Autodesk Fusion 360 part; units mm, degrees
sketch "Sketch1" plane through (0, 0, 0) normal (0, 0, 1) x (1, 0, 0)
  circle A0 centre (0, 0) radius 1.65
  circle A1 centre (0, 0) radius 3.65
  line L0 (0, 0) -> (0, -3.65)
  line L1 (0, 0) -> (0, 3.65)
  line L2 (0, 3.65) -> (15, 3.65)
  line L3 (0, -3.65) -> (15, -3.65)
  line L4 (0, 1.65) -> (12.4019, 1.65)
  line L5 (0, -1.65) -> (12.4019, -1.65)
  line L6 (16.5, 2.15) -> (16.5, 1.65)
  line L7 (16.5, -2.15) -> (16.5, -1.65)
  arc A2 (15, -0.15) -> (13.701, -0.9) centre (15, -1.65) ccw
  arc A3 (16.5, -1.65) -> (15, -0.15) centre (15, -1.65) ccw
  arc A4 (13.701, 0.9) -> (15, 0.15) centre (15, 1.65) ccw
  arc A5 (15, 0.15) -> (16.5, 1.65) centre (15, 1.65) ccw
  arc A6 (13.701, 0.9) -> (12.4019, 1.65) centre (12.4019, 0.15) ccw
  arc A7 (12.4019, -1.65) -> (13.701, -0.9) centre (12.4019, -0.15) ccw
  arc A8 (15, -3.65) -> (16.5, -2.15) centre (15, -2.15) ccw
  arc A9 (16.5, 2.15) -> (15, 3.65) centre (15, 2.15) ccw
  point P0 (16.5, 3.65)
  point P1 (16.5, -3.65)
  point P2 (13.5, 1.65)
  point P3 (13.5, -1.65)
  point P4 (16.5, 3.65)
  point P5 (16.5, 0.15)
  point P6 (16.5, -3.65)
  point P7 (16.5, -0.15)
  point P8 (13.5, 0.15)
  point P9 (13.5, -0.15)
  dimension "d1" = 3.3
  dimension "d2" = 7.3
  dimension "d10" = 16.5
  dimension "d11" = 16.5
  dimension "d18" = 13.5
  dimension "d19" = 13.5
  dimension "d23" = 3.5
  dimension "d24" = 3.5
  dimension "d25" = 3
  dimension "d26" = 3
  dimension "d27" = 1.5
  dimension "d28" = 1.5
  dimension "d29" = 1.5
  dimension "d30" = 1.5
  dimension "d31" = 1.5
  dimension "d32" = 1.5
  dimension "d33" = 1.5
  dimension "d34" = 1.5
extrude "Extrude4" add sketch "Sketch1" along normal blind 6 contours A0 A1 L0 L1 | A1 L1 L4 | A1 L0 L5 | A1 L2 L4 L6 A4 A5 A6 A9 | A1 L3 L5 L7 A2 A3 A7 A8
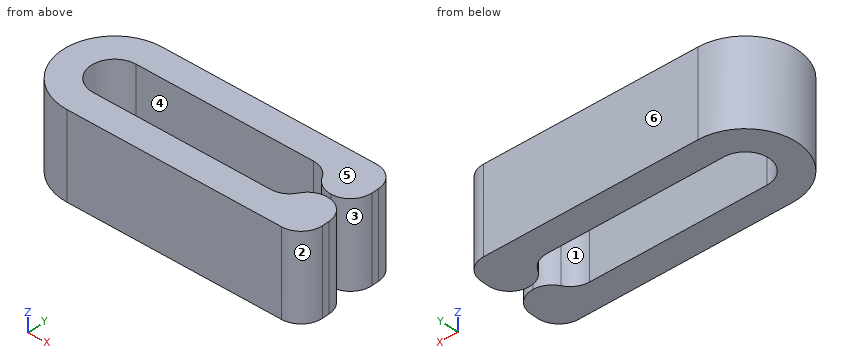
Part model, mm, in its own coordinate system. Face numbers are marked on the shaded views. A direction names the side the tool comes from. Coordinates: 2 decimals unless noted, no trailing zeros. Write each loop counter-clockwise with the first axis right and the second up, starting at its lowest first coordinate (ties: lowest second). Pieces come first, ordered by that corner, then holes. Notation, with made-up numbers: M 54.25,59 L 80.25,59 A19 ccw 80.25,65 Z; hole C 72,66.25 d8. An arc over 180 degrees is marked long. Return JSON: item names as keys, results as strings.
1. Pull direction Y, two halves, no side cores. Call the marked faces 4, 5 and 6: pulls with the +Y half, pulls with the -Y half, needs draft (parallel to the pull), parting line crosses it, or undercut.
Determined:
{"face 4": "undercut", "face 5": "needs draft", "face 6": "pulls with the +Y half"}
2. Saw through at C-C, the plane y = -0.5. Write the cut outline in (x, z).
Determined:
{"outline": "M -3.62,0 L -1.57,0 L -1.57,6 L -3.62,6 Z; M 14.04,0 L 15.96,0 L 15.96,6 L 14.04,6 Z"}
3. Saw through at B-B, the plane z = 5.15. Write the cut outline in (x, y).
Determined:
{"outline": "M 0,-3.65 L 15,-3.65 A1.5 ccw 16.5,-2.15 L 16.5,-1.65 A1.5 ccw 15,-0.15 A1.5 ccw 13.7,-0.9 A1.5 cw 12.4,-1.65 L 0,-1.65 A1.65 cw 0,1.65 L 12.4,1.65 A1.5 cw 13.7,0.9 A1.5 ccw 15,0.15 A1.5 ccw 16.5,1.65 L 16.5,2.15 A1.5 ccw 15,3.65 L 0,3.65 A3.65 ccw Z"}
4. Flat gauge pin, fed straight in: pin 1 Ø3 at (y, z) = (1, 3.5) entering from -X. Where does the tip first touch, or does it go through?
Determined:
{"pin 1": "x = -3.65"}
5. Probe L1, parallel to Y at x = 9.5, z = 4.65; L2, parallel to X at y = -1.5, z = 0.5; L3, parallel to X at y = 3, z = 5.1. List the from-to ranges inside material, lowest first.
Determined:
{"L1": "-3.65 to -1.65, 1.65 to 3.65", "L2": "-3.33 to -0.69, 13.06 to 16.49", "L3": "-2.08 to 16.24"}
6. Saw through at A-A, the plane x = 8.5. Write the cut outline in (y, z).
Determined:
{"outline": "M -3.65,0 L -1.65,0 L -1.65,6 L -3.65,6 Z; M 1.65,0 L 3.65,0 L 3.65,6 L 1.65,6 Z"}
7. 3-axis set-ups, long thin cutter, end or side, ignore diameter. For the marked faces 1, 2 and 3: which of +Z, -Z, +X, -X, +Y, -Y reach the whole face in a straight line?
Determined:
{"face 1": "+Z, -Z", "face 2": "+Z, -Z, +X, -Y", "face 3": "+Z, -Z, +X"}
8. Saw through at D-D, the plane y = 2.75. Write the cut outline in (x, z).
Determined:
{"outline": "M -2.4,0 L 16.37,0 L 16.37,6 L -2.4,6 Z"}
